Verification items for the finished model (mm, model axes). A direction names the side the tool comes from. Round coordinates to 2 decimals unless told otherwise and drop trailing zeros. Write each loop counter-clockwise with the first axis right and the second up, starting at its lowest first coordinate (ties: lowest second). Pieces come first, ordered by that corner, then holes. Notation, with made-up numbers: M -6,51.25 L 15,51.25 A25 ccw 15,69.25 Z; hole C 71,38.25 d8. An arc over 180 degrees is marked long. Answer in a Markdown table with one row per item. Add a question column.
1. Sectioned sample at D-D on x = -17.5. Record the cut outline in (y, z), plus the area to 3 significant figures.
2. Draft check along Z on faces 1 (the flat face through (0, -12, 16)), 2 (the flat face through (12, -11.432, 11)), 3 (the cylindrical face through (-21.06, -0.16, 15.49)), 4 (the cylindrical face through (-16, 0, 52)). Enter one of: pulls with the +Z half, pulls with the -Z half, needs draft (parallel to the pull), parting line crosses it, or undercut.
3. Set-up check for faces 5 (the flat face through (-12, -11.432, 11)), 6 (the cylindrical face through (5.999, -11.533, 6.11)), 7 (the flat face through (11, 0, 43)), 8 (the flat face through (0, 12, 16)): record each of +Z, -Z, +X, -X, +Y, -Y from which the full face is reachable in a straight line by a thin tool's end or side.
4. Sectioned sample at A-A on y = -7. Record the cut outline in (x, z), plus the area to 3 significant figures.
5. Sectioned sample at B-B on x = 1. Record the cut outline in (y, z), plus the area to 3 significant figures.
6. Go/stop test with flat-tipped pins: pin 1 Ø6 at (x, z) = (11.5, 9.5) entering from -Y; pin 2 Ø5 at (x, y) = (-3.5, 3) entering from -Z; pin 3 Ø1.5 at (x, z) = (18, 51) entering from -Y; pin 4 Ø1 at (x, y) = (16.5, -2.5) entering from +Z. Record where each tip stops, or that it passes through.
7. Sectioned sample at C-C on z = 15. Record the cut outline in (x, y), plus the area to 3 significant figures.
8. Material ranges on probe 1 along X at (y, z) = (6, 57); probe 2 along Y at (x, z) = (-18, 57); probe 3 along Y at (x, z) = (0, 7), recorded low to high.
```python
from build123d import *
from build123d.topology import SkipClean

# Parameters (mm, degrees)
SKETCH1_R                = 13
BOSS_EXTRUDE1_DEPTH      = 16
BOSS_EXTRUDE2_DEPTH      = 11.431752
BOSS_EXTRUDE2_DEPTH_BACK = 11.431752
CUT_EXTRUDE1_DEPTH       = 73.346389042
CUT_EXTRUDE1_DEPTH_BACK  = 73.346389042
CUT_EXTRUDE2_DEPTH       = 73.346389042
CUT_EXTRUDE2_DEPTH_BACK  = 73.346389042
SKETCH4_R                = 5
CUT_EXTRUDE3_DEPTH       = 73.346389042
CUT_EXTRUDE3_DEPTH_BACK  = 73.346389042
SKETCH5_R                = 9


with BuildPart() as part:
    # Sketch1 → Boss-Extrude1 (new body)
    with BuildSketch(Plane.XY):
        Circle(SKETCH1_R)
    extrude(amount=BOSS_EXTRUDE1_DEPTH)

    # Sketch2 → Boss-Extrude2 (add, two sides: drawn at the far end of the back side and taken through both)
    with BuildSketch(Plane(origin=(0, 0, 0), x_dir=(1, 0, 0), z_dir=(0, 1, 0)).offset(-BOSS_EXTRUDE2_DEPTH_BACK)):
        with BuildLine():
            Line((-11, -27), (-11, -67))
            Line((-11, -67), (-19.088617564, -67))
            Line((-19.088617564, -67), (-24, -27))
            ThreePointArc((-24, -27), (-16.970562748, -10.029437252), (0, -3))
            ThreePointArc((0, -3), (16.970562748, -10.029437252), (24, -27))
            Line((24, -27), (19.088617564, -67))
            Line((19.088617564, -67), (11, -67))
            Line((11, -67), (11, -27))
            ThreePointArc((11, -27), (7.778174593, -19.221825407), (0, -16))
            ThreePointArc((0, -16), (-7.778174593, -19.221825407), (-11, -27))
        make_face()
    extrude(amount=BOSS_EXTRUDE2_DEPTH + BOSS_EXTRUDE2_DEPTH_BACK)

    # Sketch3 → Cut-Extrude1 (cut, two sides: drawn at the far end of the back side and taken through both)
    with BuildSketch(Plane(origin=(0, 0, 0), x_dir=(0, 0, -1), z_dir=(1, 0, 0)).offset(-CUT_EXTRUDE1_DEPTH_BACK)):
        with BuildLine():
            ThreePointArc((-67, 0), (-64.071067812, 7.071067812), (-57, 10))
            Line((-57, 10), (-16, 11.431751549))
            Line((-16, 11.431751549), (-16, 13))
            Line((-16, 13), (-67, 13))
            Line((-67, 13), (-67, 0))
        make_face()
        with BuildLine():
            ThreePointArc((-57, -10), (-64.071067812, -7.071067812), (-67, 0))
            Line((-67, 0), (-67, -13))
            Line((-67, -13), (-16, -13))
            Line((-16, -13), (-16, -11.431751549))
            Line((-16, -11.431751549), (-57, -10))
        make_face()
    extrude(amount=CUT_EXTRUDE1_DEPTH + CUT_EXTRUDE1_DEPTH_BACK, mode=Mode.SUBTRACT)

    # Sketch4 → Cut-Extrude2 (cut, two sides: drawn at the far end of the back side and taken through both)
    with BuildSketch(Plane(origin=(0, 0, 0), x_dir=(0, 0, -1), z_dir=(1, 0, 0)).offset(-CUT_EXTRUDE2_DEPTH_BACK)):
        with Locations(Location((-57, 0, 0), (0, 0, 180))):
            Circle(SKETCH4_R)
    extrude(amount=CUT_EXTRUDE2_DEPTH + CUT_EXTRUDE2_DEPTH_BACK, mode=Mode.SUBTRACT)

    # Sketch5 → Cut-Extrude3 (cut, two sides: drawn at the far end of the back side and taken through both)
    with SkipClean():  # the faces are left unmerged after this step: merging them gives an invalid solid
        with BuildSketch(Plane(origin=(0, 0, 0), x_dir=(-1, 0, 0), z_dir=(0, 0, -1)).offset(-CUT_EXTRUDE3_DEPTH_BACK)):
            Circle(SKETCH5_R)
        extrude(amount=CUT_EXTRUDE3_DEPTH + CUT_EXTRUDE3_DEPTH_BACK, mode=Mode.SUBTRACT)


solid = part.part
```
Geometry check:
| question | item | result |
|---|---|---|
| 1 | outline | M -11.43,10.58 L 11.43,10.58 L 11.43,16 L 10,57 A10 ccw -10,57 L -11.43,16 Z; hole C 0,57 d10 |
| 1 | area | 1,080 mm2 |
| 2 | face 1 | pulls with the +Z half |
| 2 | face 2 | needs draft |
| 2 | face 3 | pulls with the -Z half |
| 2 | face 4 | undercut |
| 3 | face 5 | +Z, -Z, -X, -Y |
| 3 | face 6 | -Z |
| 3 | face 7 | +Z, +Y, -Y |
| 3 | face 8 | +Z, +X, -X, +Y |
| 4 | outline | M -24,27 A24 ccw -10.95,5.65 L -10.95,0 L -5.66,0 L -5.66,17.57 A11 cw -11,27 L -11,64.14 L -19.44,64.14 Z; M 5.66,0 L 10.95,0 L 10.95,5.65 A24 ccw 24,27 L 19.44,64.14 L 11,64.14 L 11,27 A11 cw 5.66,17.57 Z |
| 4 | area | 1,410 mm2 |
| 5 | outline | M -12.96,0 L -8.94,0 L -8.94,16.05 L -11.43,16.05 L -11.43,16 L -12.96,16 Z; M 8.94,0 L 12.96,0 L 12.96,16 L 11.43,16 L 11.43,16.05 L 8.94,16.05 Z |
| 5 | area | 129 mm2 |
| 6 | pin 1 | stops at y = -11.43 |
| 6 | pin 2 | passes through |
| 6 | pin 3 | stops at y = -10.24 |
| 6 | pin 4 | stops at z = 66.8 |
| 7 | outline | M -20.78,-11.43 L -6.19,-11.43 A13 ccw 6.19,-11.43 L 20.78,-11.43 L 20.78,11.43 L 6.19,11.43 A13 ccw -6.19,11.43 L -20.78,11.43 Z; hole C 0,0 d18 |
| 7 | area | 722 mm2 |
| 8 | probe 1 | x = -20.32 to -11, 11 to 20.32 |
| 8 | probe 2 | y = -10 to -5, 5 to 10 |
| 8 | probe 3 | y = -13 to -9, 9 to 13 |
